Could you check a few things on this model? Use its own coordinates, in mm. A direction names the side the tool comes from. Give positions to 0.01 mm unless a question says otherwise; leave off trailing zeros. Order: outer loops, then holes, each group sorted by start corner. A loop starts at its lowest first (then second) coordinate and runs counter-clockwise, first axis right, second up. Notation, with made-up numbers: (32.25, 49) -> (84.25, 49) arc R17 cw to (84.25, 78) -> close; hole circle Ø1 at (87, 82.5). An arc over 180 degrees is marked (long way). Write each question's results on one line, items separated by ' | '.
```python
from build123d import *

# Parameters (mm, degrees)
SKETCH1_R                   = 10.2489
BOSS_EXTRUDE1_DEPTH         = 2.9845
BOSS_EXTRUDE1_2_DEPTH       = 2.9845
SKETCH2_R                   = 10.2489
BOSS_EXTRUDE2_DEPTH         = 5.08
BOSS_EXTRUDE3_DEPTH         = 3.81
F_1_4_0_25_DIAMETER_HOLE1_D = 6.35
BOSS_EXTRUDE4_DEPTH         = 17.78
SKETCH8_R                   = 2.25
CUT_EXTRUDE1_DEPTH          = 17.78
SKETCH9_W                   = 17.78
SKETCH9_H                   = 2.54
BOSS_EXTRUDE5_DEPTH         = 17.78
CUT_EXTRUDE2_REACH          = 251.039
CUT_EXTRUDE3_DEPTH          = 20
BOSS_EXTRUDE6_DEPTH         = 2.54
BOSS_EXTRUDE7_DEPTH         = 39.624
CUT_EXTRUDE5_DEPTH          = 6.35
F_6_CLEARANCE_HOLE1_D       = 3.7973
SKETCH19_W                  = 39.624
SKETCH19_H                  = 13.560471889
BOSS_EXTRUDE8_DEPTH         = 6.35
M4_CLEARANCE_HOLE1_D        = 4.5
SKETCH20_R                  = 4.308
CUT_EXTRUDE6_DEPTH          = 195.822050963
FILLET1_R                   = 11
CUT_EXTRUDE7_DEPTH          = 6.35


with BuildPart() as part:
    # Sketch1 → Boss-Extrude1 (new body)
    with BuildSketch(Plane.XY):
        Circle(SKETCH1_R)
    extrude(amount=BOSS_EXTRUDE1_DEPTH)



with BuildPart() as body_2:
    # Sketch1 → Boss-Extrude1 2 (new body)
    with BuildSketch(Plane.XY):
        with Locations((-72.411066703, 81.765798589)):
            Circle(SKETCH1_R)
    extrude(amount=BOSS_EXTRUDE1_2_DEPTH)


with BuildPart() as part_1:
    add(part.part)

    add(body_2.part)  # Boss-Extrude2 merges body 2
    # Sketch2 → Boss-Extrude2 (add)
    with BuildSketch(Plane.XY.offset(2.9845)):
        with Locations((-72.411066703, 81.765798589)):
            Circle(SKETCH2_R)
        Circle(SKETCH2_R)
    extrude(amount=BOSS_EXTRUDE2_DEPTH)

    # Sketch3 → Boss-Extrude3 (add)
    with BuildSketch(Plane.XY.offset(8.0645)):
        Polygon((-134.069705847, 103.500499391), (-96.039101852, 137.180065299), (52.150988145, -30.154592279), (14.12038415, -63.834158187), align=None)
    extrude(amount=BOSS_EXTRUDE3_DEPTH)

    # 1/4 (0.25) Diameter Hole1 (through all)
    with Locations(Plane.XY.offset(11.8745)):
        with Locations((0, 0), (-72.411066703, 81.765798589)):
            Hole(F_1_4_0_25_DIAMETER_HOLE1_D / 2)

    # Sketch7 → Boss-Extrude4 (add)
    with BuildSketch(Plane(origin=(0, 0, 8.0645), x_dir=(-1, 0, 0), z_dir=(0, 0, -1))):
        Polygon((53.34482504, 12.346831233), (66.604496657, 27.319509971), (61.850671158, 31.529455709), (48.59099954, 16.556776971), align=None)
        Polygon((120.810034229, 88.527820652), (134.069705847, 103.500499391), (129.315880348, 107.710445129), (116.05620873, 92.737766391), align=None)
    extrude(amount=BOSS_EXTRUDE4_DEPTH)

    # Sketch8 → Cut-Extrude1 (cut)
    with BuildSketch(Plane(origin=(-19.015301997, -16.839782954, 0), x_dir=(0, 0, -1), z_dir=(0.7486339369082552, 0.6629835808745542, 0))):
        with Locations(Location((0.8255, 54.61, 0), (0, 0, 90))):
            Circle(SKETCH8_R)
        with Locations(Location((0.8255, 156.37, 0), (0, 0, 90))):
            Circle(SKETCH8_R)
    extrude(amount=-CUT_EXTRUDE1_DEPTH, mode=Mode.SUBTRACT)

    # Sketch9 → Boss-Extrude5 (add)
    with BuildSketch(Plane(origin=(-19.015301997, -16.839782954, 0), x_dir=(0, 0, -1), z_dir=(0.7486339369082552, 0.6629835808745542, 0))):
        with Locations((0.8255, 63.34)):
            Rectangle(SKETCH9_W, SKETCH9_H)
        with Locations((0.8255, 45.88)):
            Rectangle(SKETCH9_W, SKETCH9_H)
        with Locations((0.8255, 165.1)):
            Rectangle(SKETCH9_W, SKETCH9_H)
        with Locations((0.8255, 147.64)):
            Rectangle(SKETCH9_W, SKETCH9_H)
    extrude(amount=BOSS_EXTRUDE5_DEPTH)

    # Cut-Extrude2: up to this face of the body (flat: up to its plane)
    cut_extrude2_end = Plane(part_1.part.faces().sort_by_distance((-111.777765781, 96.526717556, -0.8255))[0])
    # Sketch10 → Cut-Extrude2 (cut, up to the picked face)
    with BuildSketch(Plane(origin=(-110.30057835, 124.550228083, 0), x_dir=(0.7486339369082557, 0.6629835808745536, 0), z_dir=(-0.6629835808745536, 0.7486339369082557, 0)), mode=Mode.PRIVATE) as cut_extrude2_sk1:
        Polygon((-7.62, 9.7155), (-7.62, -8.0645), (-25.4, 9.7155), align=None)
    cut_extrude2_tool1 = split(extrude(cut_extrude2_sk1.sketch, amount=-CUT_EXTRUDE2_REACH, mode=Mode.PRIVATE), bisect_by=cut_extrude2_end, keep=Keep.BOTH, mode=Mode.PRIVATE)
    add(cut_extrude2_tool1.solids().sort_by(Axis((-120.442073, 115.569011, -3.788833), (0.6629835808745536, -0.7486339369082557, 0)))[0], mode=Mode.SUBTRACT)

    # Sketch11 → Cut-Extrude3 (cut)
    with BuildSketch(Plane(origin=(-42.83536916, 48.369238664, 0), x_dir=(0.7486339369082559, 0.6629835808745536, 0), z_dir=(-0.6629835808745536, 0.7486339369082559, 0))):
        Polygon((-7.62, 9.7155), (-7.62, -8.0645), (-25.4, 9.7155), align=None)
    extrude(amount=-CUT_EXTRUDE3_DEPTH, mode=Mode.SUBTRACT)

    # Sketch13 → Boss-Extrude6 (add)
    with BuildSketch(Plane(origin=(-110.30057835, 124.550228083, 0), x_dir=(0.7486339369082557, 0.6629835808745536, 0), z_dir=(-0.6629835808745536, 0.7486339369082557, 0))):
        Polygon((-25.4, 9.7155), (19.05, 9.7155), (19.05, -8.0645), (-7.62, -8.0645), align=None)
    extrude(amount=-BOSS_EXTRUDE6_DEPTH)

    # Sketch14 → Boss-Extrude7 (add)
    with BuildSketch(Plane(origin=(0, 0, 8.0645), x_dir=(-1, 0, 0), z_dir=(0, 0, -1))):
        Polygon((-52.150988145, -30.154592279), (-14.12038415, -63.834158187), (-5.700492673, -54.326507188), (-43.731096668, -20.64694128), align=None)
    extrude(amount=BOSS_EXTRUDE7_DEPTH)

    # Sketch15 → Cut-Extrude5 (cut)
    with BuildSketch(Plane.XY.offset(11.8745)):
        Polygon((38.433391408, -33.820658256), (42.550325055, -30.174738298), (37.334398928, -28.432329153), (33.21746528, -32.078249111), (33.824088825, -35.052507224), align=None)
        Polygon((43.649317536, -35.563067402), (43.042693991, -32.588809289), (38.433391408, -33.820658256), (34.31645776, -37.466578215), (39.532383888, -39.20898736), align=None)
        Polygon((38.433391408, -33.820658256), (43.042693991, -32.588809289), (42.550325055, -30.174738298), align=None)
        Polygon((34.31645776, -37.466578215), (38.433391408, -33.820658256), (33.824088825, -35.052507224), align=None)
        Polygon((21.198191786, -46.233889763), (19.41808941, -50.660441211), (23.535023058, -47.014521252), align=None)
        Polygon((15.301155763, -54.306361169), (17.637987035, -55.086992658), (19.41808941, -50.660441211), align=None)
        Polygon((14.202163283, -48.918032065), (15.301155763, -54.306361169), (19.41808941, -50.660441211), (21.198191786, -46.233889763), (18.31909693, -45.272112107), align=None)
        Polygon((19.41808941, -50.660441211), (17.637987035, -55.086992658), (20.51708189, -56.048770314), (24.634015538, -52.402850356), (23.535023058, -47.014521252), align=None)
    extrude(amount=-CUT_EXTRUDE5_DEPTH, mode=Mode.SUBTRACT)

    # #6 Clearance Hole1 (through all)
    with Locations(Plane.XY.offset(5.5245)):
        with Locations((19.41808941, -50.660441211), (38.433391408, -33.820658256)):
            Hole(F_6_CLEARANCE_HOLE1_D / 2)

    # Sketch19 → Boss-Extrude8 (add)
    with BuildSketch(Plane(origin=(-23.769127497, -21.049728693, 0), x_dir=(0, 0, 1), z_dir=(-0.7486339369082559, -0.6629835808745536, 0))):
        with Locations((-11.7475, -37.669764056)):
            Rectangle(SKETCH19_W, SKETCH19_H)
    extrude(amount=-BOSS_EXTRUDE8_DEPTH)

    # M4 Clearance Hole1 (through all)
    with Locations(Plane(origin=(-19.015301997, -16.839782954, 0), x_dir=(0, 0, -1), z_dir=(0.7486339369082555, 0.6629835808745539, 0))):
        with Locations((1.866346616, -40.889528111), (21.728039849, -40.889528111)):
            Hole(M4_CLEARANCE_HOLE1_D / 2)

    # Sketch20 → Cut-Extrude6 (cut, through all)
    with BuildSketch(Plane(origin=(-19.015301997, -16.839782954, 0), x_dir=(0, 0, -1), z_dir=(0.7486339369082555, 0.6629835808745539, 0))):
        with Locations((21.728039849, -40.889528111)):
            Circle(SKETCH20_R)
        with Locations((1.866346616, -40.889528111)):
            Circle(SKETCH20_R)
    extrude(amount=CUT_EXTRUDE6_DEPTH, mode=Mode.SUBTRACT)

    # Fillet1
    # the kernel refuses this fillet: 11 mm, written as the material it adds along each edge
    with BuildSketch(Plane(origin=(-127.631902052, 105.808914929, 8.0645), x_dir=(0.6629835808745532, -0.7486339369082561, 1.2918958832001814e-15), z_dir=(0.7486339369082562, 0.6629835808745532, 0))) as fillet1_piece_1:
        with BuildLine():
            CenterArc((FILLET1_R, FILLET1_R), FILLET1_R, 180, 90)
            Line((0, FILLET1_R), (0, 0))
            Line((0, 0), (FILLET1_R, 0))
        make_face()
    extrude(amount=44.45)
    # the kernel refuses this fillet: 11 mm, written as the material it takes off along each edge
    with BuildSketch(Plane(origin=(-154.657139112, 85.268450917, 11.8745), x_dir=(0, 0, -1), z_dir=(0.7486339369082557, 0.6629835808745537, 0))) as fillet1_2_piece_1:
        with BuildLine():
            CenterArc((FILLET1_R, -FILLET1_R), FILLET1_R, 90, 90)
            Line((0, -FILLET1_R), (0, 0))
            Line((0, 0), (FILLET1_R, 0))
        make_face()
    extrude(amount=105.8, mode=Mode.SUBTRACT)
    with BuildSketch(Plane(origin=(72.73842141, -11.922543805, 11.8745), x_dir=(-0.6629835808745536, 0.7486339369082557, 0), z_dir=(-0.7486339369082559, -0.6629835808745537, 0))) as fillet1_2_piece_2:
        with BuildLine():
            CenterArc((FILLET1_R, FILLET1_R), FILLET1_R, 180, 90)
            Line((0, FILLET1_R), (0, 0))
            Line((0, 0), (FILLET1_R, 0))
        make_face()
    extrude(amount=105.8, mode=Mode.SUBTRACT)

    # Sketch23 → Cut-Extrude7 (cut)
    with BuildSketch(Plane.XY.offset(5.5245)):
        Polygon((37.334398928, -28.432329153), (33.21746528, -32.078249111), (34.31645776, -37.466578215), (39.532383888, -39.20898736), (43.649317536, -35.563067402), (42.550325055, -30.174738298), align=None)
        Polygon((14.202163283, -48.918032065), (15.301155763, -54.306361169), (20.51708189, -56.048770314), (24.634015538, -52.402850356), (23.535023058, -47.014521252), (18.31909693, -45.272112107), align=None)
    extrude(amount=-CUT_EXTRUDE7_DEPTH, mode=Mode.SUBTRACT)


solid = part_1.part
```
Q1. For faces 1 (the cylindrical face through (27.355, -36.148, -21.692)), 2 (the flat face through (39.979, -29.316, 5.613)), 3 (the flat face through (-75, 84, 0)), 4 (the flat face through (-2.4, 2.4, 0)), 5 (the cylindrical face through (-2.222, -10.005, 3.976)), which set-ups out of +Z, -Z, +X, -X, +Y, -Y let a thin tool reach every point of the face, with its end or its side?
Here are the results:
face 1: +Y | face 2: +Z | face 3: -Z, +X, +Y | face 4: -Z, +X, -X, +Y | face 5: -Z
Q2. I need wall thicknesses on line 1 along Y through (x, z) = (0, 4.75) (3 decimals); line 2 along Z through (x, y) = (29.5, -11.5); line 3 along Y through (x, z) = (27, -4). Which ranges of each line are inside material? Lowest first, please.
Here are the results:
line 1: y = -47.89 to -41.261, -10.249 to -3.175, 3.175 to 10.249 | line 2: z = 8.06 to 11.87 | line 3: y = -52.43 to -35.71
Q3. Suppose I cut it at A-A on y = 0. Please give me the cut outline in (x, z) (1 decimal), and give its area (3 significant figures).
Here are the results:
outline: (-42.4, 8.1) -> (-10.2, 8.1) -> (-10.2, 0) -> (-3.2, 0) -> (-3.2, 11.9) -> (-42.4, 11.9) -> close; (3.2, 0) -> (10.2, 0) -> (10.2, 8.1) -> (25.4, 8.1) -> (25.4, 11.9) -> (3.2, 11.9) -> close | area: 348 mm²
Q4. Suppose I cut it at B-B on z = -15. Please give me the cut outline in (x, y), and give its area (3 significant figures).
Here are the results:
outline: (-3.29, -44.17) -> (14.12, -63.83) -> (52.15, -30.15) -> (43.73, -20.65) -> (10.45, -50.12) -> (1.46, -39.96) -> close; hole circle Ø3.8 at (19.42, -50.66); hole circle Ø3.8 at (38.43, -33.82) | area: 709 mm²
Q5. Thinking about a two-plate mould opening in X: for faces 6 (the cylindrical face through (0.69, -3.1, 5.85)), 7 (the flat face through (-47, 37, 11.875)), 8 (the cylindrical face through (-113.241, 117.756, 8.567)), 9 (the flat face through (14.744, -51.574, 5.613)), which applies, +X half, -X half, draft (parallel to the pull), parting line (faces both ways), or undercut?
Here are the results:
face 6: undercut | face 7: draft | face 8: -X half | face 9: undercut
Q6. I'm going to push flat-ended pins straight in: pin 1 Ø6 at (x, y) = (38.43, -33.82) entering from +Z; pin 2 Ø6 at (x, y) = (-68.5, 86) entering from -Z; pin 3 Ø14.5 at (x, y) = (-53.5, 25) entering from -Z. Where does each tip first touch, or does it pass through?
Here are the results:
pin 1: stops at z = -0.83 | pin 2: stops at z = 0 | pin 3: stops at z = -9.72
